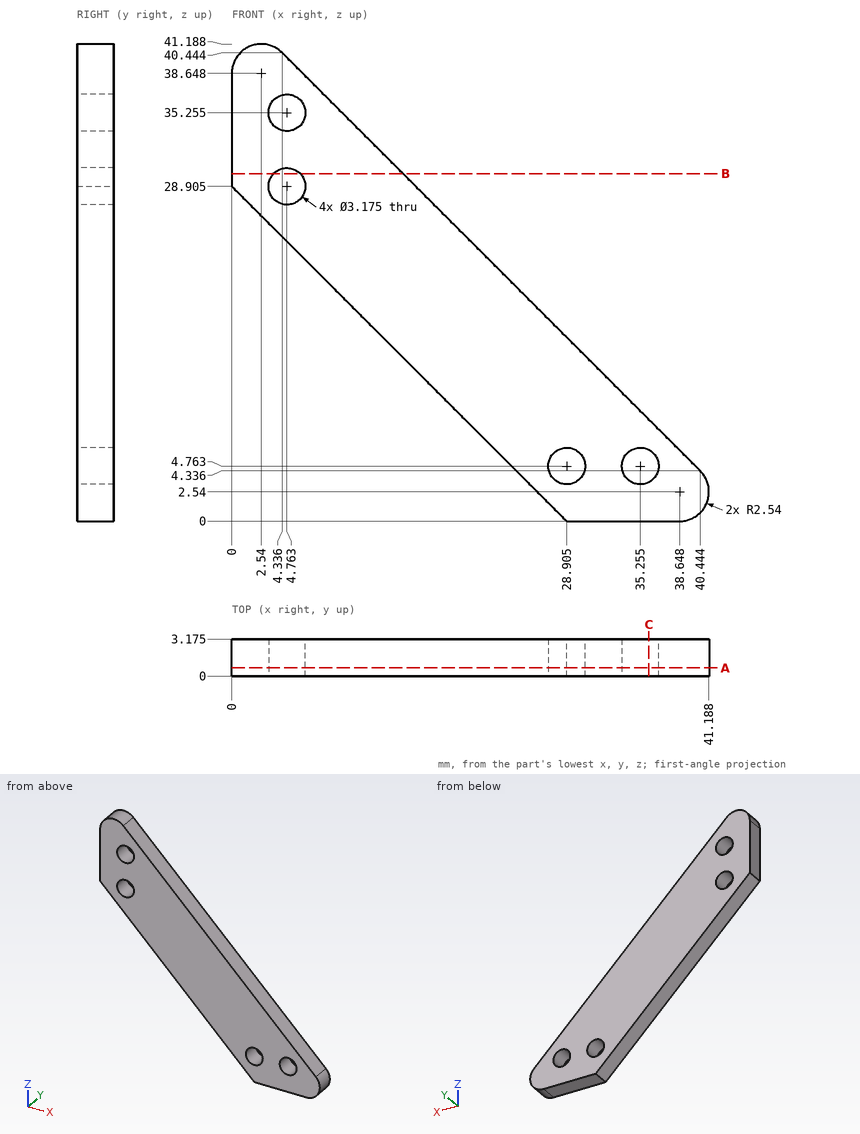
Answer from the drawing. Dimensions are ordinates in mm from the lowest x, y and z of the part. Give positions to 0.01 mm unless a question says otherwise; leave off trailing zeros. Write each loop counter-clockwise with the first axis right and the second up, starting at its lowest first coordinate (ties: lowest second). Pieces come first, ordered by that corner, then holes.
1) Given P1, Ø3.5, axis at x = 4.76, z = 35.26, coming from the +Y side (1 decimal), flat-ended and moving along its own axis, determine where the tip first touches the part or whether it passes through.
2) Section C-C (x = 36) is taken. Write down the section's boundary in (y, z) (1 decimal), and give its area (3 significant figures).
3) Section A-A (y = 0.7) is taken. Count the separate pieces of the cut face and the enclosed holes in it, and give its area (3 significant figures).
4) Find the intervals of material crossed by L1, parallel to X at y = 2.8, z = 4.5 (1 decimal); L2, parallel to X at y = 1.35, z = 35.5 (1 decimal); L3, parallel to X at y = 0.2, z = 7 (1 decimal), in increasing order.
5) Section B-B (z = 30) is taken. Write down the section's boundary in (x, y) (1 decimal).
Response:
1. P1: stops at y = 3.2
2. outline: (0, 0) - (3.2, 0) - (3.2, 3.4) - (0, 3.4) - close; (0, 6.2) - (3.2, 6.2) - (3.2, 8.8) - (0, 8.8) - close
2. area: 19.0 mm2
3. separate pieces: 1
3. enclosed holes: 4
3. area: 537 mm2
4. L1: x = 24.4 to 27.3, 30.5 to 33.7, 36.8 to 40.3
4. L2: x = 0 to 3.2, 6.3 to 9.3
4. L3: x = 21.9 to 37.8
5. outline: (0, 0) - (3.6, 0) - (3.6, 3.2) - (0, 3.2) - close; (5.9, 0) - (14.8, 0) - (14.8, 3.2) - (5.9, 3.2) - close
